Source: CAD feature listing. Evaluate the final solid. Frame: model axes, mm. A direction names the side the tool comes from. Give positions to 0.01 mm unless a question says otherwise; leave off trailing zeros. Order: outer loops, then holes, each group sorted by start corner. A loop starts at its lowest first (then second) coordinate and runs counter-clockwise, first axis right, second up. Notation, with made-up numbers: (-35, 17) -> (-3, 17) arc R31 cw to (-3, 41) -> close; hole circle Ø9 at (37.25, 4). An arc over 180 degrees is marked (long way). Use CSV: the item, a comma, the result in double quotes.
```python
from build123d import *

# Parameters (mm, degrees)
EXTRUDE_THIN1_DEPTH = 174.625
FILLET1_R           = 1.27


with BuildPart() as part:
    # Sketch1 → Extrude-Thin1 (new body)
    with BuildSketch(Plane.XY):
        with BuildLine():
            Line((0, 0), (-12.7, 0))
            Line((-12.7, 0), (-12.7, 3.175))
            ThreePointArc((-12.7, 3.175), (-14.094903955, 6.542596045), (-17.4625, 7.9375))
            Line((-17.4625, 7.9375), (-17.4625, 12.7))
            Line((-17.4625, 12.7), (-16.1925, 12.7))
            Line((-16.1925, 12.7), (-16.1925, 9.07230076))
            ThreePointArc((-16.1925, 9.07230076), (-12.769295804, 6.965104303), (-11.43, 3.175))
            Line((-11.43, 3.175), (-11.43, 1.27))
            Line((-11.43, 1.27), (0, 1.27))
            Line((0, 1.27), (0, 0))
        make_face()
    extrude(amount=-EXTRUDE_THIN1_DEPTH)

    # Fillet1
    fillet1_edges = [part.edges().sort_by_distance(p)[0] for p in [
        (-12.7, 0, -87.3125),
        (-17.4625, 7.9375, -87.3125),
    ]]
    fillet(fillet1_edges, radius=FILLET1_R)


solid = part.part
```
1. Section query A-A on z = -15. Return loops of the section in (x, y) (1 decimal), plus the area to 3 significant figures.
Answer below:
outline,"(-17.5, 9.1) arc R1.3 ccw to (-16.5, 7.8) arc R4.8 cw to (-12.7, 3.2) -> (-12.7, 1.3) arc R1.3 ccw to (-11.4, 0) -> (0, 0) -> (0, 1.3) -> (-11.4, 1.3) -> (-11.4, 3.2) arc R6 ccw to (-16.2, 9.1) -> (-16.2, 12.7) -> (-17.5, 12.7) -> close"
area,"33.2 mm²"
2. Ray query, line 1 along X through (y, z) = (12.25, -44.5); line 2 along Y through (x, z) = (-16.5, -154.5); line 3 along X through (y, z) = (3.75, -114). Return the intervals inside material, ascending.
Answer below:
line 1,"x = -17.46 to -16.19"
line 2,"y = 7.84 to 12.7"
line 3,"x = -12.73 to -11.46"
3. Section query C-C on y = 11.25. Return loops of the section in (x, z) (1 decimal).
Answer below:
outline,"(-17.5, -174.6) -> (-16.2, -174.6) -> (-16.2, 0) -> (-17.5, 0) -> close"
4. Access query for faces 1 (the flat face through (-6, 1.27, -86)), 2 (the flat face through (-17.462, 11, -86)). Directions: +Z, -Z, +X, -X, +Y, -Y. A direction counts if a zero-diameter tool reaches every point of the face in a straight line with its end or side. Return the directions, or none.
Answer below:
face 1,"+Z, -Z, +X, +Y"
face 2,"+Z, -Z, -X, +Y, -Y"
5. Pin query (flat end, axial travel): P1, Ø1.5, axis at x = -8, y = 1.5, coming from the +Z side; P2, Ø5, axis at x = -12, z = -113.5, coming from the +Y side; P3, Ø3, axis at y = 11, z = -56.5, coming from the +X side; P4, Ø1, axis at y = 2, z = -50, coming from the -X side. Return the tip coordinate at first contact, or that it passes through.
Answer below:
P1,"stops at z = 0"
P2,"stops at y = 8.43"
P3,"stops at x = -16.19"
P4,"stops at x = -12.7"
6. Section query B-B on x = -3. Return loops of the section in (y, z) (3 decimals), plus the area to 3 significant figures.
Answer below:
outline,"(0, -174.625) -> (1.27, -174.625) -> (1.27, 0) -> (0, 0) -> close"
area,"222 mm²"
